Can you work these out from the model? Positions are in its coordinate system, mm. Face numbers are marked on the shaded views. A direction names the side the tool comes from. Round coordinates to 2 decimals unless told otherwise and drop trailing zeros. Order: outer loops, then holes, each group sorted by start corner. A loop starts at its lowest first (then second) coordinate and runs counter-clockwise, first axis right, second up.
from build123d import *

# Parameters (mm, degrees)
BOSS_EXTRUDE1_DEPTH  = 7.5
M4_CLEARANCE_HOLE1_D = 4.5
M2_CLEARANCE_HOLE1_D = 2.4


with BuildPart() as part:
    # Sketch1 → Boss-Extrude1 (new body, symmetric)
    with BuildSketch(Plane.XY):
        with BuildLine():
            Line((0, 0), (22.225, 0))
            Line((22.225, 0), (22.225, 20.569946809))
            Line((22.225, 20.569946809), (19.05, 20.569946809))
            Line((19.05, 20.569946809), (19.05, 6.175))
            ThreePointArc((19.05, 6.175), (18.171320344, 4.053679656), (16.05, 3.175))
            Line((16.05, 3.175), (6.175, 3.175))
            ThreePointArc((6.175, 3.175), (4.053679656, 4.053679656), (3.175, 6.175))
            Line((3.175, 6.175), (3.175, 20))
            Line((3.175, 20), (0, 20))
            Line((0, 20), (0, 0))
        make_face()
    extrude(amount=BOSS_EXTRUDE1_DEPTH, both=True)

    # M4 Clearance Hole1 (through all)
    with Locations(Plane(origin=(0, 3.175, 0), x_dir=(1, 0, 0), z_dir=(0, 1, 0))):
        with Locations((11.1125, -4.5), (11.1125, 4.5)):
            Hole(M4_CLEARANCE_HOLE1_D / 2)

    # M2 Clearance Hole1 (through all)
    with Locations(Plane.ZY):
        with Locations((0, 15)):
            Hole(M2_CLEARANCE_HOLE1_D / 2)


solid = part.part
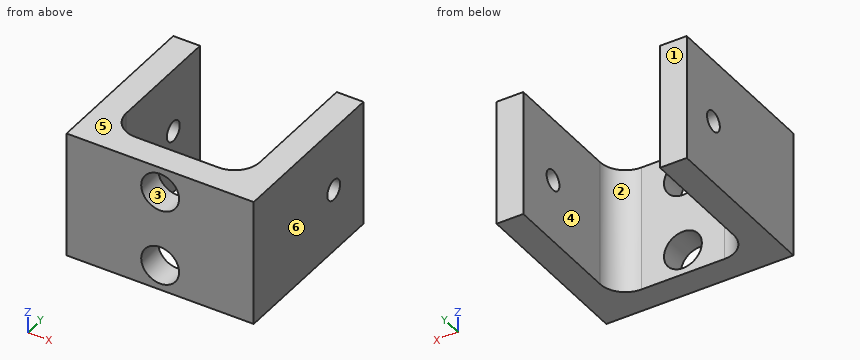
(1) I'm going to push flat-ended pins straight in: pin 1 Ø4 at (x, z) = (11.11, -4.5) entering from -Y; pin 2 Ø3 at (x, z) = (10.5, -1) entering from +Y (3 decimals); pin 3 Ø1 at (x, z) = (1, 1.5) entering from +Y. Where does each tip first touch, or does it pass through?
(2) Please list where these lines run through material, in increasing order: probe 1 along X at (y, z) = (13.5, -4) (3 decimals); probe 2 along Y at (x, z) = (2.1, 0); probe 3 along Y at (x, z) = (21.05, 0).
(3) I want a section at C-C, the plane z = 0. List the corners of the cut face in (x, y) for me (3 decimals), plus the area to 3 significant figures.
(4) On a 3-axis mill with a long thin cutter (end or side, diameter ignored), from which of +Z, -Z, +X, -X, +Y, -Y can I reach the whole of each face in a straight line? I mean the marked faces 1, 2 and 3. Say none if no direction works.
(5) If we mould it in two halves opening along X, with no side actions, what happens to the marked faces 4, 5 and 6? For each: pulls with the +X half, pulls with the -X half, needs draft (parallel to the pull), parting line crosses it, or undercut.
(6) I want a section at D-D, the plane y = 2.5. Give the number of separate pieces and of enclosed holes in the cut face, plus the area to 3 significant figures.
(7) I want a section at A-A, the plane y = 18.5. List the corners of the cut face in (x, z) for me (3 decimals).
Ans:
1. pin 1: passes through
1. pin 2: stops at y = 3.175
1. pin 3: stops at y = 20
2. probe 1: x = 0 to 3.175, 19.05 to 22.225
2. probe 2: y = 0 to 13.8, 16.2 to 20
2. probe 3: y = 0 to 13.8, 16.2 to 20.57
3. outline: (0, 0) - (22.225, 0) - (22.225, 13.8) - (19.05, 13.8) - (19.05, 6.175) arc R3 cw to (16.05, 3.175) - (6.175, 3.175) arc R3 cw to (3.175, 6.175) - (3.175, 13.8) - (0, 13.8) - close; (0, 16.2) - (3.175, 16.2) - (3.175, 20) - (0, 20) - close; (19.05, 16.2) - (22.225, 16.2) - (22.225, 20.57) - (19.05, 20.57) - close
3. area: 168 mm2
4. face 1: +Z, -Z, -X, +Y
4. face 2: +Z, -Z, +Y
4. face 3: +Y, -Y
5. face 4: undercut
5. face 5: needs draft
5. face 6: pulls with the +X half
6. separate pieces: 1
6. enclosed holes: 2
6. area: 302 mm2
7. outline: (0, -7.5) - (3.175, -7.5) - (3.175, 7.5) - (0, 7.5) - close; (19.05, -7.5) - (22.225, -7.5) - (22.225, 7.5) - (19.05, 7.5) - close
